```python
from build123d import *

# Parameters (mm, degrees)
SKETCH1_W                    = 409
SKETCH1_H                    = 20
BOSS_EXTRUDE1_DEPTH          = 3.175
CSK_FOR_M4_SFHCS1_AT_2_COUNT = 2
CSK_FOR_M4_SFHCS1_AT_2_PITCH = 14.142135624
CSK_FOR_M4_SFHCS1_AT_3_COUNT = 2
CSK_FOR_M4_SFHCS1_AT_3_PITCH = 10
CSK_FOR_M4_SFHCS1_AT_4_COUNT = 2
CSK_FOR_M4_SFHCS1_AT_4_PITCH = 10
CSK_FOR_M4_SFHCS1_AT_5_COUNT = 2
CSK_FOR_M4_SFHCS1_AT_5_PITCH = 390
CSK_FOR_M4_SFHCS1_AT_6_COUNT = 2
CSK_FOR_M4_SFHCS1_AT_6_PITCH = 390.128184063
M4X0_7_TAPPED_HOLE1_D        = 3.3


with BuildPart() as part:
    # Sketch1 → Boss-Extrude1 (new body)
    with BuildSketch(Plane(origin=(0, 0, 0), x_dir=(1, 0, 0), z_dir=(0, 1, 0))):
        Rectangle(SKETCH1_W, SKETCH1_H)
    extrude(amount=BOSS_EXTRUDE1_DEPTH)

    # Sketch4 → CSK for M4 SFHCS1 (revolve, cut)
    with BuildSketch(Plane(origin=(-190, 3.175, -5), x_dir=(0, 0, 1), z_dir=(1, 0, 0))):
        Polygon((0, 0), (0, 3.175), (2.25, 3.175), (2.25, 2.23), (4.48, 0), align=None)
    csk_for_m4_sfhcs1 = revolve(axis=Axis((-190, 9.525, -5), (0, -1, 0)), mode=Mode.SUBTRACT)

    # CSK for M4 SFHCS1 at 2: CSK for M4 SFHCS1 ×2
    with Locations(*[Vector(-0.7071067811865472, 0, 0.7071067811865479) * (i * CSK_FOR_M4_SFHCS1_AT_2_PITCH) for i in range(1, CSK_FOR_M4_SFHCS1_AT_2_COUNT)]):
        add(csk_for_m4_sfhcs1, mode=Mode.SUBTRACT)

    # CSK for M4 SFHCS1 at 3: CSK for M4 SFHCS1 ×2
    with Locations(*[(-i * CSK_FOR_M4_SFHCS1_AT_3_PITCH, 0, 0) for i in range(1, CSK_FOR_M4_SFHCS1_AT_3_COUNT)]):
        add(csk_for_m4_sfhcs1, mode=Mode.SUBTRACT)

    # CSK for M4 SFHCS1 at 4: CSK for M4 SFHCS1 ×2
    with Locations(*[(0, 0, i * CSK_FOR_M4_SFHCS1_AT_4_PITCH) for i in range(1, CSK_FOR_M4_SFHCS1_AT_4_COUNT)]):
        add(csk_for_m4_sfhcs1, mode=Mode.SUBTRACT)

    # CSK for M4 SFHCS1 at 5: CSK for M4 SFHCS1 ×2
    with Locations(*[(i * CSK_FOR_M4_SFHCS1_AT_5_PITCH, 0, 0) for i in range(1, CSK_FOR_M4_SFHCS1_AT_5_COUNT)]):
        add(csk_for_m4_sfhcs1, mode=Mode.SUBTRACT)

    # CSK for M4 SFHCS1 at 6: CSK for M4 SFHCS1 ×2
    with Locations(*[Vector(0.9996714309094813, 0, 0.025632600792550815) * (i * CSK_FOR_M4_SFHCS1_AT_6_PITCH) for i in range(1, CSK_FOR_M4_SFHCS1_AT_6_COUNT)]):
        add(csk_for_m4_sfhcs1, mode=Mode.SUBTRACT)

    # M4x0.7 Tapped Hole1 (through all)
    with Locations(Plane(origin=(0, 3.175, 0), x_dir=(1, 0, 0), z_dir=(0, 1, 0))):
        with Locations((100, 5), (-100, -5), (-100, 5), (100, -5)):
            Hole(M4X0_7_TAPPED_HOLE1_D / 2)


solid = part.part
```
Geometry check sheet. Reference: the model listing, model coordinates, mm. Round coordinates to 2 decimals unless told otherwise and drop trailing zeros. Use a Markdown table: item, result. Add a question column.
1) Mould release check, pull along Z, two halves, no side actions. Record for faces 1 (the conical face through (-197.67, 1.08, -5.52)), 2 (the flat face through (-3, 3.175, 0)), 3 (the conical face through (202.33, 1.08, -5.52)): released by +Z, released by -Z, zero draft, split by the parting line, or undercut.
2) Thickness scan on line 1 along X through (y, z) = (0.9, 5); line 2 along Z through (x, y) = (-200, 0.55); line 3 along X through (y, z) = (1, -5) (3 decimals). Record the ranges inside material, lowest first.
3) Gauge pin test, flat end, axial feed: P1, Ø7, axis at x = -200, z = 5, coming from the +Y side (3 decimals). Record the tip position at first contact, or that the pin passes through.
4) Section check A-A (y = 1.6). Count the separate pieces of the cut face and the enclosed holes in it, then the cut area to 3 significant figures.
Established:
| question | item | result |
|---|---|---|
| 1 | face 1 | undercut |
| 1 | face 2 | zero draft |
| 1 | face 3 | undercut |
| 2 | line 1 | -204.5 to -202.25, -197.75 to -192.25, -187.75 to -101.65, -98.35 to 98.35, 101.65 to 197.75, 202.25 to 204.5 |
| 2 | line 2 | -10 to -7.25, -2.75 to 2.75, 7.25 to 10 |
| 2 | line 3 | -204.5 to -202.305, -197.695 to -192.305, -187.695 to -101.65, -98.35 to 98.35, 101.65 to 197.695, 202.305 to 204.5 |
| 3 | P1 | y = 2.195 |
| 4 | separate pieces | 1 |
| 4 | enclosed holes | 10 |
| 4 | area | 7,990 mm2 |
